Verification items for the finished model (mm, model axes). A direction names the side the tool comes from. Give positions to 0.01 mm unless a question says otherwise; leave off trailing zeros. Loops run counter-clockwise (first coordinate to the right, second up) from the corner with the lowest first, then second, coordinate; pieces in that order, holes last. Notation, with made-up numbers: M -19.5,-37 L 34.5,-37 A27 cw 34.5,-16 Z; hole C 10.25,25 d6. An arc over 180 degrees is marked long. Use CSV: the item, a comma, the result in double quotes.
Autodesk Inventor part; units mm, degrees
ref_plane "YZ Plane" through (0, 0, 0) normal (1, 0, 0) x (0, 1, 0)
ref_plane "XZ Plane" through (0, 0, 0) normal (0, 1, 0) x (-1, 0, 0)
ref_plane "XY Plane" through (0, 0, 0) normal (0, 0, 1) x (1, 0, 0)
sketch "Sketch1" plane through (0, 0, 0) normal (0, 1, 0) x (-1, 0, 0)
  line L0 (0, 0) -> (30, 0)
  line L1 (30, 0) -> (30, -25)
  line L2 (30, -25) -> (0, -25)
  line L3 (0, -25) -> (0, 0)
  dimension "d0" = 30
  dimension "d1" = 25
extrude "Extrusion1" add sketch "Sketch1" along normal blind 20
sketch "Sketch2" plane through (0, 0, 0) normal (0, -1, 0) x (1, 0, 0)
  circle A0 centre (-20, -12.5) radius 2.5
  line L0 (0, 0) -> (0, -25)
  point P0 (0, -12.5)
  dimension "d4" = 5
  dimension "d15" = 20
extrude "Extrusion2" cut sketch "Sketch2" against normal blind 5
sketch "Sketch3" plane through (0, 0, 0) normal (1, 0, 0) x (0, 0, -1)
  line L0 (17.5, 7.5) -> (7.5, 7.5)
  line L1 (7.5, 7.5) -> (7.5, 12.5)
  line L2 (7.5, 12.5) -> (17.5, 12.5)
  line L3 (17.5, 12.5) -> (17.5, 7.5)
  line L4 (17.5, 7.5) -> (7.5, 12.5) construction
  line L5 (7.5, 7.5) -> (17.5, 12.5) construction
  point P0 (0, 0)
  point P1 (12.5, 10)
  dimension "d7" = 10
  dimension "d8" = 5
extrude "Extrusion3" add sketch "Sketch3" along normal blind 9
sketch "Sketch4" plane through (0, 12.5, -7.5) normal (0, 1, 0) x (1, 0, 0)
  circle A0 centre (5, 5) radius 2.5
  line L0 (0, -7.5) -> (0, 17.5)
  dimension "d11" = 5
  dimension "d14" = 5
extrude "Extrusion4" cut sketch "Sketch4" against normal through all
properties part number "head"
(1) Mould release check, pull along Z, two halves, no side actions. Record for faces 1 (the flat face through (9, 10, -12)), 2 (the flat face through (4, 10, -17.5)), 3 (the flat face through (-20, 5, -12)), 4 (the cylindrical face through (-22, 2, -14)): released by +Z, released by -Z, zero draft, split by the parting line, or undercut.
Calculated:
face 1,"zero draft"
face 2,"released by -Z"
face 3,"undercut"
face 4,"undercut"
(2) Section check A-A on x = 5. Record the cut outline in (y, z).
Calculated:
outline,"M 7.5,-17.5 L 12.5,-17.5 L 12.5,-15 L 7.5,-15 Z; M 7.5,-10 L 12.5,-10 L 12.5,-7.5 L 7.5,-7.5 Z"
(3) Tool access check on faces 5 (the flat face through (-15, 20, -12)), 6 (the flat face through (2, 12.5, -12)), 7 (the flat face through (2, 7.5, -13)), 8 (the flat face through (4, 10, -7.5)). Record the directions out of +Z, -Z, +X, -X, +Y, -Y that give a thin tool (end or side, any length) a straight path to the whole face; none if there is none.
Calculated:
face 5,"+Z, -Z, +X, -X, +Y"
face 6,"+Z, -Z, +X, +Y"
face 7,"+Z, -Z, +X, -Y"
face 8,"+Z, +X, +Y, -Y"
(4) Depth check by flat-ended pin: pin 1 Ø2.5 at (x, z) = (-19.5, -12) entering from -Y; pin 2 Ø5 at (x, z) = (-11, -22) entering from -Y; pin 3 Ø1.5 at (x, y) = (6, 9.5) entering from -Z; pin 4 Ø1.5 at (y, z) = (17.5, -4) entering from +X. Enter the tip coordinate at first touch or a pass-through.
Calculated:
pin 1,"stops at y = 5"
pin 2,"stops at y = 0"
pin 3,"stops at z = -17.5"
pin 4,"stops at x = 0"
(5) Scan lines: L1, parallel to Z at x = -20, y = 1.9; L2, parallel to X at y = 10.65, z = -12.5; L3, parallel to Z at x = 5, y = 9.05. Record each from-to range of solid material in increasing order. Write a range as from..to.
Calculated:
L1,"z = -25..-15, -10..0"
L2,"x = -30..2.5, 7.5..9"
L3,"z = -17.5..-15, -10..-7.5"
(6) Section check B-B on z = -12.5. Record the cut outline in (x, y).
Calculated:
outline,"M -30,0 L -22.5,0 L -22.5,5 L -17.5,5 L -17.5,0 L 0,0 L 0,7.5 L 2.5,7.5 L 2.5,12.5 L 0,12.5 L 0,20 L -30,20 Z; M 7.5,7.5 L 9,7.5 L 9,12.5 L 7.5,12.5 Z"
(7) Section check C-C on y = 3.5. Record the cut outline in (x, z), plus the area to 3 significant figures.
Calculated:
outline,"M -30,-25 L 0,-25 L 0,0 L -30,0 Z; hole C -20,-12.5 d5"
area,"730 mm²"
(8) Section check D-D on x = -20. Record the cut outline in (y, z).
Calculated:
outline,"M 0,-25 L 20,-25 L 20,0 L 0,0 L 0,-10 L 5,-10 L 5,-15 L 0,-15 Z"
